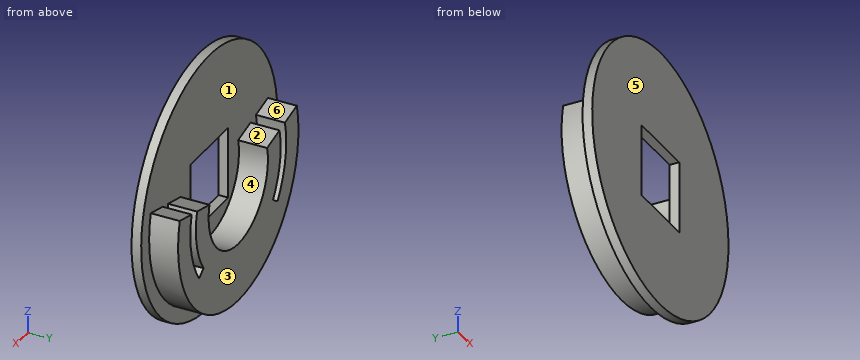
```python
from build123d import *

# Parameters (mm, degrees)
BOSS_EXTRUDE1_DEPTH = 6
SKETCH2_R           = 27
SKETCH2_W           = 15
SKETCH2_H           = 15
BOSS_EXTRUDE2_DEPTH = 2
CUT_EXTRUDE1_DEPTH  = 6


with BuildPart() as part:
    # Sketch1 → Boss-Extrude1 (new body)
    with BuildSketch(Plane(origin=(0, 0, 0), x_dir=(1, 0, 0), z_dir=(0, 1, 0))):
        with BuildLine():
            Line((-23.207164842, -5.5), (-11.433299241, -2.709643606))
            ThreePointArc((-11.433299241, -2.709643606), (0, 11.75), (11.433299241, -2.709643606))
            Line((11.433299241, -2.709643606), (23.207164842, -5.5))
            ThreePointArc((23.207164842, -5.5), (0, 23.85), (-23.207164842, -5.5))
        make_face()
    extrude(amount=BOSS_EXTRUDE1_DEPTH)

    # Sketch2 → Boss-Extrude2 (add)
    with BuildSketch(Plane.XZ):
        with Locations(Location((0, 0, 0), (0, 0, 270))):
            Circle(SKETCH2_R)
        Rectangle(SKETCH2_W, SKETCH2_H, mode=Mode.SUBTRACT)
    extrude(amount=BOSS_EXTRUDE2_DEPTH)

    # Sketch3 → Cut-Extrude1 (cut)
    with BuildSketch(Plane(origin=(0, 6, 0), x_dir=(1, 0, 0), z_dir=(0, 1, 0))):
        with BuildLine():
            Line((-15.555508902, 10.909910303), (-13.754344713, 9.646657531))
            ThreePointArc((-13.754344713, 9.646657531), (-16.499364166, 3.16401361), (-16.347185297, -3.874213836))
            Line((-16.347185297, -3.874213836), (-18.487888134, -4.381551363))
            ThreePointArc((-18.487888134, -4.381551363), (-18.659995187, 3.578348726), (-15.555508902, 10.909910303))
        make_face()
    cut_extrude1 = extrude(amount=-CUT_EXTRUDE1_DEPTH, mode=Mode.SUBTRACT)

    # Mirror1: Cut-Extrude1 across plane
    add(cut_extrude1.mirror(Plane(origin=(0, 0, 0), x_dir=(0, 0, 1), z_dir=(1, 0, 0))), mode=Mode.SUBTRACT)


solid = part.part
```
Input: part model. Units: mm. Frame: model coordinates. Face numbers are marked on the shaded views. A direction names the side the tool comes from. Coordinates: 2 decimals unless noted, no trailing zeros. Loops run counter-clockwise (first coordinate to the right, second up) from the corner with the lowest first, then second, coordinate; pieces in that order, holes last. Notation, with made-up numbers: M 48.5,10 L 105.5,10 A25 cw 105.5,42 Z; hole C -35.75,-35 d11. An arc over 180 degrees is marked long. Answer in a Markdown table with one row per item.
1. Section A-A, the plane z = 0. Output: boundary loops of the cut face in (x, y), then the cut area to 3 significant figures.
Response:
| item | result |
|---|---|
| outline | M -27,-2 L -7.5,-2 L -7.5,0 L -11.75,0 L -11.75,6 L -16.8,6 L -16.8,0 L -19,0 L -19,6 L -23.85,6 L -23.85,0 L -27,0 Z; M 7.5,-2 L 27,-2 L 27,0 L 23.85,0 L 23.85,6 L 19,6 L 19,0 L 16.8,0 L 16.8,6 L 11.75,6 L 11.75,0 L 7.5,0 Z |
| area | 197 mm2 |
2. Section B-B, the plane x = 0. Output: boundary loops of the cut face in (y, z).
Response:
| item | result |
|---|---|
| outline | M -2,-27 L 0,-27 L 0,-23.85 L 6,-23.85 L 6,-11.75 L 0,-11.75 L 0,-7.5 L -2,-7.5 Z; M -2,7.5 L 0,7.5 L 0,27 L -2,27 Z |
3. Section D-D, the plane z = -18.5. Output: boundary loops of the cut face in (x, y), then the cut area to 3 significant figures.
Response:
| item | result |
|---|---|
| outline | M -19.67,-2 L 19.67,-2 L 19.67,0 L 15.05,0 L 15.05,6 L -15.05,6 L -15.05,0 L -19.67,0 Z |
| area | 259 mm2 |
4. Reachability of the marked faces 1, 2 and 3 from +Z, -Z, +X, -X, +Y, -Y: full face, straight path, thin tool, end or side. Return the list, or none.
Response:
| item | result |
|---|---|
| face 1 | +Y |
| face 2 | +Z, +Y |
| face 3 | +Z, -Z, +X, -X, +Y |
5. Draft query along Z for the marked faces 4, 5 and 6. Return one class per face: pulls with the +Z half, pulls with the -Z half, needs draft (parallel to the pull), parting line crosses it, or undercut.
Response:
| item | result |
|---|---|
| face 4 | undercut |
| face 5 | needs draft |
| face 6 | pulls with the +Z half |
6. First-contact query: pin 1 (2 mm diameter, centred on y = -1, z = 3, fed in from -X); pin 2 (10 mm diameter, centred on x = 14.5, z = 7, fed in from +Y); pin 3 (0.6 mm diameter, centred on x = 1, y = -1, fed in from +Z); pin 4 (0.6 mm diameter, centred on y = -1, z = -3.5, fed in from +X). Flat tips, straight axial feed; report the tip coordinate or a pass-through.
Response:
| item | result |
|---|---|
| pin 1 | stops at x = -26.93 |
| pin 2 | stops at y = 6 |
| pin 3 | stops at z = 26.99 |
| pin 4 | stops at x = 26.81 |
7. Section C-C, the plane y = 2.25. Output: boundary loops of the cut face in (x, z).
Response:
| item | result |
|---|---|
| outline | M -23.21,5.5 A23.85 ccw long 23.21,5.5 L 18.49,4.38 A19 cw 15.56,-10.91 L 13.75,-9.65 A16.8 ccw 16.35,3.87 L 11.43,2.71 A11.75 cw long -11.43,2.71 L -16.35,3.87 A16.8 ccw -13.75,-9.65 L -15.56,-10.91 A19 cw -18.49,4.38 Z |
8. Material intervals for line 1 (X direction, y = 3.3, z = 0); line 2 (X direction, y = 1.75, z = 2.5); line 3 (Y direction, x = -0.5, z = -24), sorted ascending.
Response:
| item | result |
|---|---|
| line 1 | x = -23.85 to -19, -16.8 to -11.75, 11.75 to 16.8, 19 to 23.85 |
| line 2 | x = -23.72 to -18.83, -16.61 to -11.48, 11.48 to 16.61, 18.83 to 23.72 |
| line 3 | y = -2 to 0 |
